from build123d import *

# Parameters (mm, degrees)
BOSS_EXTRUDE1_DEPTH  = 4
CUT_EXTRUDE2_DEPTH   = 10
SKETCH4_W            = 270
SKETCH4_H            = 4.5
CUT_EXTRUDE5_DEPTH   = 10
CUT_EXTRUDE6_DEPTH   = 10
MIRROR9_COPY_1_DEPTH = 10
CHAMFER1_SIZE        = 10
SKETCH6_R            = 2.25
CUT_EXTRUDE7_DEPTH   = 10
SKETCH7_R            = 2.25
CUT_EXTRUDE8_DEPTH   = 10


with BuildPart() as part:
    # Sketch1 → Boss-Extrude1 (new body)
    with BuildSketch(Plane.XY):
        Polygon((440.319741737, -451.518776284), (440.319741737, -431.518776284), (430.319741737, -421.518776284), (310.319741737, -421.518776284), (210.319741737, -421.518776284), (90.319741737, -421.518776284), (80.319741737, -431.518776284), (80.319741737, -451.518776284), (70.319741737, -461.518776284), (2.319741737, -461.518776284), (-29.680258263, -461.518776284), (-39.680258263, -451.518776284), (-39.680258263, -421.518776284), (-39.680258263, -5.004819249), (-39.680258263, 98.481223716), (0.319741737, 98.481223716), (540.319741737, 98.481223716), (560.319741737, 98.481223716), (560.319741737, -5.004819249), (560.319741737, -420.004819249), (560.319741737, -451.518776284), (550.319741737, -461.518776284), (540.319741737, -461.518776284), (450.319741737, -461.518776284), align=None)
    extrude(amount=BOSS_EXTRUDE1_DEPTH)

    # Sketch3 → Cut-Extrude2 (cut)
    with BuildSketch(Plane(origin=(0, 0, 0), x_dir=(-1, 0, 0), z_dir=(0, 0, -1))):
        Polygon((-410.319741737, -391.518776284), (-420.319741737, -391.518776284), (-430.319741737, -381.518776284), (-430.319741737, 8.481223716), (-420.319741737, 18.481223716), (-410.319741737, 18.481223716), align=None)
        Polygon((-100.319741737, 18.481223716), (-90.319741737, 8.481223716), (-90.319741737, -381.518776284), (-100.319741737, -391.518776284), (-110.319741737, -391.518776284), (-110.319741737, 18.481223716), align=None)
    extrude(amount=-CUT_EXTRUDE2_DEPTH, mode=Mode.SUBTRACT)

    # Sketch4 → Cut-Extrude5 (cut)
    with BuildSketch(Plane(origin=(0, 0, 0), x_dir=(-1, 0, 0), z_dir=(0, 0, -1))):
        with Locations((-255.319741737, -106.429112329)):
            Rectangle(SKETCH4_W, SKETCH4_H)
    extrude(amount=-CUT_EXTRUDE5_DEPTH, mode=Mode.SUBTRACT)

    # Sketch5 → Cut-Extrude6 (cut)
    with BuildSketch(Plane(origin=(0, 0, 0), x_dir=(-1, 0, 0), z_dir=(0, 0, -1))):
        Polygon((-171.743467553, -99.679112329), (-260.319741737, -99.679112329), (-260.319741737, -95.179112329), (-173.607428584, -95.179112329), (-138.607428584, -60.179112329), (-125.319741737, -60.179112329), (-125.319741737, -64.679112329), (-136.743467553, -64.679112329), align=None)
    cut_extrude6 = extrude(amount=-CUT_EXTRUDE6_DEPTH, mode=Mode.SUBTRACT)

    # Mirror3: Cut-Extrude6 across plane
    add(cut_extrude6.mirror(Plane(origin=(260.319741737, -99.679112329, 10), x_dir=(0, 0, 1), z_dir=(1, 0, 0))), mode=Mode.SUBTRACT)

    # Mirror9: Cut-Extrude6 across plane
    add(cut_extrude6.mirror(Plane(origin=(0, -106.429112329, 0), x_dir=(0, 0, 1), z_dir=(0, -1, 0))), mode=Mode.SUBTRACT)

    # Mirror9 copy 1 sketch → Mirror9 copy 1 (cut)
    with BuildSketch(Plane(origin=(520.639483474, -212.858224657, 0), x_dir=(1, 0, 0), z_dir=(0, 0, -1))):
        Polygon((-171.743467553, -99.679112329), (-260.319741737, -99.679112329), (-260.319741737, -95.179112329), (-173.607428584, -95.179112329), (-138.607428584, -60.179112329), (-125.319741737, -60.179112329), (-125.319741737, -64.679112329), (-136.743467553, -64.679112329), align=None)
    extrude(amount=-MIRROR9_COPY_1_DEPTH, mode=Mode.SUBTRACT)

    # Chamfer1
    chamfer1_edges = [part.edges().sort_by_distance(p)[0] for p in [
        (-39.680258263, 98.481223716, 2),
        (560.319741737, 98.481223716, 2),
    ]]
    chamfer(chamfer1_edges, length=CHAMFER1_SIZE)

    # Sketch6 → Cut-Extrude7 (cut)
    with BuildSketch(Plane(origin=(0, 0, 0), x_dir=(-1, 0, 0), z_dir=(0, 0, -1))):
        with Locations((-540.319741737, 48.481223716)):
            Circle(SKETCH6_R)
        with Locations((-540.319741737, -111.518776284)):
            Circle(SKETCH6_R)
        with Locations((-540.319741737, -271.518776284)):
            Circle(SKETCH6_R)
        with Locations((-540.319741737, -431.518776284)):
            Circle(SKETCH6_R)
    cut_extrude7 = extrude(amount=-CUT_EXTRUDE7_DEPTH, mode=Mode.SUBTRACT)

    # Mirror10: Cut-Extrude7 across plane
    add(cut_extrude7.mirror(Plane(origin=(260.319741737, 0, 0), x_dir=(0, 0, 1), z_dir=(1, 0, 0))), mode=Mode.SUBTRACT)

    # Sketch7 → Cut-Extrude8 (cut)
    with BuildSketch(Plane.XY.offset(4)):
        with Locations((65.604902337, 88.481223716)):
            Circle(SKETCH7_R)
        with Locations((95.604902337, 88.481223716)):
            Circle(SKETCH7_R)
        with Locations((95.604902337, 68.481223716)):
            Circle(SKETCH7_R)
        with Locations((65.604902337, 68.481223716)):
            Circle(SKETCH7_R)
    cut_extrude8 = extrude(amount=-CUT_EXTRUDE8_DEPTH, mode=Mode.SUBTRACT)

    # Mirror11: Cut-Extrude8 across plane
    add(cut_extrude8.mirror(Plane(origin=(260.319741737, 0, 0), x_dir=(0, 0, 1), z_dir=(1, 0, 0))), mode=Mode.SUBTRACT)


solid = part.part
Could you check a few things on this model? Use its own coordinates, in mm. A direction names the side the tool comes from. Coordinates: 2 decimals unless noted, no trailing zeros. Order: outer loops, then holes, each group sorted by start corner. A loop starts at its lowest first (then second) coordinate and runs counter-clockwise, first axis right, second up. Notation, with made-up numbers: (77, 71.25) - (116, 71.25) arc R26 ccw to (116, 86.25) - close; hole circle Ø8 at (36, 52.5). An arc over 180 degrees is marked (long way). Answer in a Markdown table with one row per item. Add a question column.
(1) If we mould it in two halves opening along X, with no side actions, what happens to faces 3 (the face through (265, -178, 0)), 4 (the face through (366.641, -81.934, 1.972)), 5 (the face through (153.998, -81.934, 1.972))? For each: released by +X, released by -X, zero draft, split by the parting line, or undercut.
(2) I need wall thicknesses on L1, parallel to Y at x = 315, z = 0.7; L2, parallel to Y at x = 131, z = 2.4; L3, parallel to X at y = -168, z = 1.45. Which ranges of each line are inside material? Lowest first, please.
(3) If we section it at D-D, the plane x = 356.5: Please give me the cut outline in (y, z), then the cut area to 3 significant figures.
(4) On a 3-axis mill with a long thin cutter (end or side, diameter ignored), from which of +Z, -Z, +X, -X, +Y, -Y can I reach the whole of each face in a straight line? I mean faces 1 (the face through (156.35, -77.92, 1.97)), 2 (the face through (265, -178, 4)). Say none if no direction works.
(5) If we section it at A-A, the plane y = -237: Please give me the cut outline in (x, z), then the cut area to 3 significant figures.
(6) If we section it at B-B, the plane x = 238: Please give me the cut outline in (y, z).
(7) If we section it at C-C, the plane y = -133.5: Please give me the cut outline in (x, z), then the cut area to 3 significant figures.
(8) Will this pin go through, and if not, where does the flat tip stop? pin 1 (1.2 mm diameter, centred on x = 235.5, z = 3, fed in from -Y).
Results are:
| question | item | result |
|---|---|---|
| 1 | face 3 | zero draft |
| 1 | face 4 | undercut |
| 1 | face 5 | undercut |
| 2 | L1 | y = -421.52 to -117.68, -113.18 to -108.68, -104.18 to -99.68, -95.18 to 98.48 |
| 2 | L2 | y = -421.52 to -152.68, -148.18 to -108.68, -104.18 to -64.68, -60.18 to 98.48 |
| 2 | L3 | x = -39.68 to 90.32, 110.32 to 410.32, 430.32 to 560.32 |
| 3 | outline | (-421.52, 0) - (-127.15, 0) - (-127.15, 4) - (-421.52, 4) - close; (-120.78, 0) - (-108.68, 0) - (-108.68, 4) - (-120.78, 4) - close; (-104.18, 0) - (-92.08, 0) - (-92.08, 4) - (-104.18, 4) - close; (-85.71, 0) - (98.48, 0) - (98.48, 4) - (-85.71, 4) - close |
| 3 | area | 2,010 mm2 |
| 4 | face 1 | +Z, -Z |
| 4 | face 2 | +Z, +X, -X, +Y, -Y |
| 5 | outline | (-39.68, 0) - (90.32, 0) - (90.32, 4) - (-39.68, 4) - close; (110.32, 0) - (410.32, 0) - (410.32, 4) - (110.32, 4) - close; (430.32, 0) - (560.32, 0) - (560.32, 4) - (430.32, 4) - close |
| 5 | area | 2,240 mm2 |
| 6 | outline | (-421.52, 0) - (-117.68, 0) - (-117.68, 4) - (-421.52, 4) - close; (-113.18, 0) - (-108.68, 0) - (-108.68, 4) - (-113.18, 4) - close; (-104.18, 0) - (-99.68, 0) - (-99.68, 4) - (-104.18, 4) - close; (-95.18, 0) - (98.48, 0) - (98.48, 4) - (-95.18, 4) - close |
| 7 | outline | (-39.68, 0) - (90.32, 0) - (90.32, 4) - (-39.68, 4) - close; (110.32, 0) - (151.42, 0) - (151.42, 4) - (110.32, 4) - close; (157.79, 0) - (362.85, 0) - (362.85, 4) - (157.79, 4) - close; (369.22, 0) - (410.32, 0) - (410.32, 4) - (369.22, 4) - close; (430.32, 0) - (560.32, 0) - (560.32, 4) - (430.32, 4) - close |
| 7 | area | 2,190 mm2 |
| 8 | pin 1 | stops at y = -421.52 |
